Build history of the part. All positions in model axes, mm. A direction names the side the tool comes from. Round coordinates to 2 decimals unless told otherwise and drop trailing zeros. Write each loop counter-clockwise with the first axis right and the second up, starting at its lowest first coordinate (ties: lowest second). Pieces come first, ordered by that corner, then holes. Notation, with made-up numbers: M -6,54.5 L 51,54.5 A15 ccw 51,68.5 Z; hole C -23,11.5 d11. An arc over 180 degrees is marked long. One line per item, written item: value. Start each with the question number.
```python
from build123d import *

# Parameters (mm, degrees)
F0_DEPTH = 2.54
F1_R     = 38.1
F5_DEPTH = 2.541
F2_DEPTH = 25.4
F3_R     = 5.08


with BuildPart() as f0:
    # F4 (on Top) → F0 (new body)
    with BuildSketch(Plane.XY):
        with BuildLine():
            ThreePointArc((44.1325, 25.1587448763), (31.8906233853, 39.5427381462), (15.24, 48.460111432))
            ThreePointArc((15.24, 48.460111432), (0, 50.8), (-15.24, 48.460111432))
            ThreePointArc((-15.24, 48.460111432), (-31.8906233853, 39.5427381462), (-44.1325, 25.1587448763))
            ThreePointArc((-44.1325, 25.1587448763), (-35.0133309687, 14.0204203753), (-31.75, 0))
            Line((-31.75, 0), (31.75, 0))
            ThreePointArc((31.75, 0), (35.0133309687, 14.0204203753), (44.1325, 25.1587448763))
        make_face()
        with BuildLine():
            Line((73.025, 30.287569645), (15.24, 48.460111432))
            ThreePointArc((15.24, 48.460111432), (31.8906233853, 39.5427381462), (44.1325, 25.1587448763))
            ThreePointArc((44.1325, 25.1587448763), (57.9506836061, 31.2612793654), (73.025, 30.287569645))
        make_face()
        with BuildLine():
            ThreePointArc((-44.1325, 25.1587448763), (-31.8906233853, 39.5427381462), (-15.24, 48.460111432))
            Line((-15.24, 48.460111432), (-73.025, 30.287569645))
            ThreePointArc((-73.025, 30.287569645), (-57.9506836061, 31.2612793654), (-44.1325, 25.1587448763))
        make_face()
        with BuildLine():
            ThreePointArc((73.025, 30.287569645), (57.9506836061, 31.2612793654), (44.1325, 25.1587448763))
            ThreePointArc((44.1325, 25.1587448763), (49.1048419201, 13.0136274728), (50.8, 0))
            ThreePointArc((50.8, 0), (49.1048419201, -13.0136274728), (44.1325, -25.1587448763))
            ThreePointArc((44.1325, -25.1587448763), (57.9506836061, -31.2612793654), (73.025, -30.287569645))
            ThreePointArc((73.025, -30.287569645), (89.0976683508, -18.7835533113), (95.25, 0))
            ThreePointArc((95.25, 0), (89.0976683508, 18.7835533113), (73.025, 30.287569645))
        make_face()
        with BuildLine():
            ThreePointArc((-50.8, 0), (-49.1048419201, 13.0136274728), (-44.1325, 25.1587448763))
            ThreePointArc((-44.1325, 25.1587448763), (-57.9506836061, 31.2612793654), (-73.025, 30.287569645))
            ThreePointArc((-73.025, 30.287569645), (-95.25, 0), (-73.025, -30.287569645))
            ThreePointArc((-73.025, -30.287569645), (-57.9506836061, -31.2612793654), (-44.1325, -25.1587448763))
            ThreePointArc((-44.1325, -25.1587448763), (-49.1048419201, -13.0136274728), (-50.8, 0))
        make_face()
        with BuildLine():
            ThreePointArc((44.1325, -25.1587448763), (35.0133309687, -14.0204203753), (31.75, 0))
            Line((31.75, 0), (-31.75, 0))
            ThreePointArc((-31.75, 0), (-35.0133309687, -14.0204203753), (-44.1325, -25.1587448763))
            ThreePointArc((-44.1325, -25.1587448763), (-31.8906233853, -39.5427381462), (-15.24, -48.460111432))
            ThreePointArc((-15.24, -48.460111432), (0, -50.8), (15.24, -48.460111432))
            ThreePointArc((15.24, -48.460111432), (31.8906233853, -39.5427381462), (44.1325, -25.1587448763))
        make_face()
        with BuildLine():
            ThreePointArc((-44.1325, -25.1587448763), (-57.9506836061, -31.2612793654), (-73.025, -30.287569645))
            Line((-73.025, -30.287569645), (-15.24, -48.460111432))
            ThreePointArc((-15.24, -48.460111432), (-31.8906233853, -39.5427381462), (-44.1325, -25.1587448763))
        make_face()
        with BuildLine():
            ThreePointArc((73.025, -30.287569645), (57.9506836061, -31.2612793654), (44.1325, -25.1587448763))
            ThreePointArc((44.1325, -25.1587448763), (31.8906233853, -39.5427381462), (15.24, -48.460111432))
            Line((15.24, -48.460111432), (73.025, -30.287569645))
        make_face()
        with BuildLine():
            ThreePointArc((50.8, 0), (49.1048419201, 13.0136274728), (44.1325, 25.1587448763))
            ThreePointArc((44.1325, 25.1587448763), (35.0133309687, 14.0204203753), (31.75, 0))
            Line((31.75, 0), (50.8, 0))
        make_face()
        with BuildLine():
            ThreePointArc((44.1325, -25.1587448763), (49.1048419201, -13.0136274728), (50.8, 0))
            Line((50.8, 0), (31.75, 0))
            ThreePointArc((31.75, 0), (35.0133309687, -14.0204203753), (44.1325, -25.1587448763))
        make_face()
        with BuildLine():
            Line((-31.75, 0), (-50.8, 0))
            ThreePointArc((-50.8, 0), (-49.1048419201, -13.0136274728), (-44.1325, -25.1587448763))
            ThreePointArc((-44.1325, -25.1587448763), (-35.0133309687, -14.0204203753), (-31.75, 0))
        make_face()
        with BuildLine():
            ThreePointArc((-31.75, 0), (-35.0133309687, 14.0204203753), (-44.1325, 25.1587448763))
            ThreePointArc((-44.1325, 25.1587448763), (-49.1048419201, 13.0136274728), (-50.8, 0))
            Line((-50.8, 0), (-31.75, 0))
        make_face()
    extrude(amount=F0_DEPTH)

    # F1 (on face) → F5 (cut, through all)
    with BuildSketch(Plane.XY.offset(2.54)):
        Circle(F1_R)
    extrude(amount=-F5_DEPTH, mode=Mode.SUBTRACT)

    # F6 (on face) → F2 (join)
    with BuildSketch(Plane.XY.offset(2.54)):
        with BuildLine():
            Line((-73.025, -30.287569645), (-29.75025979, 23.8019335859))
            ThreePointArc((-29.75025979, 23.8019335859), (0, 38.1), (29.75025979, 23.8019335859))
            Line((29.75025979, 23.8019335859), (73.025, -30.287569645))
            ThreePointArc((73.025, -30.287569645), (95.25, 0), (73.025, 30.287569645))
            Line((73.025, 30.287569645), (15.24, 48.460111432))
            ThreePointArc((15.24, 48.460111432), (0, 50.8), (-15.24, 48.460111432))
            Line((-15.24, 48.460111432), (-73.025, 30.287569645))
            ThreePointArc((-73.025, 30.287569645), (-95.25, 0), (-73.025, -30.287569645))
        make_face()
    extrude(amount=F2_DEPTH)

    # F3
    f3_edges = [f0.edges().sort_by_distance(p)[0] for p in [
        (73.025, -30.28757, 15.24),
        (-73.025, -30.28757, 15.24),
        (-44.1325, 39.373841, 27.94),
        (-95.25, 0, 27.94),
        (-51.38763, -3.242818, 27.94),
        (0, 38.1, 27.94),
        (51.38763, -3.242818, 27.94),
        (95.25, 0, 27.94),
        (44.1325, 39.373841, 27.94),
        (0, 50.8, 27.94),
    ]]
    fillet(f3_edges, radius=F3_R)


solid = f0.part
```
Item 1: Cut at A-A, the plane x = 0. Write the cut outline in (y, z), plus the area to 3 significant figures.
Item 2: Two-plate mould, pull along X, no slides. Class faces 3 (the flat face through (-14, 42, 27.94)), 4 (the flat face through (-50.515, -2.152, 12.558)), 5 (the flat face through (-43.73, 39.5, 11.27)): pulls with the +X half, pulls with the -X half, needs draft (parallel to the pull), parting line crosses it, or undercut.
Item 3: Cut at C-C, the plane z = 25.75. Write the cut outline in (x, y).
Item 4: Drill centre lines: line 1 (Y direction, x = 0, z = 1.5); line 2 (X direction, y = 0, z = 1.8); line 3 (Z direction, x = 8, y = 42). Where is each one in solid material? Low to high.
Item 5: Drop flat-ended pins along their axis: pin 1 (6 mm diameter, centred on y = -10, z = 16.5, fed in from -X); pin 2 (8 mm diameter, centred on x = -73.5, y = -37.5, fed in from +Z); pin 3 (6 mm diameter, centred on x = -47.5, y = -27, fed in from +Z); pin 4 (1 mm diameter, centred on x = 74, z = 13.5, fed in from +Y). Give the stop position or say it passes through.
Item 6: Cut at B-B, the plane z = 17. Write the cut outline in (x, y) (3 decimals).
Item 7: Which spindle directions (+Z, -Z, +X, -X, +Y, -Y) get a long thin tool onto all of the face, cutting with end or side? Do faces 1 (the cylindrical face through (51.646, -1.247, 26.412)), 2 (the flat face through (44.537, 39.247, 11.27)). Say none if no direction does.
Computed values:
1. outline: M -50.8,0 L -38.1,0 L -38.1,2.54 L -50.8,2.54 Z; M 38.1,0 L 50.8,0 L 50.8,22.86 A5.08 ccw 45.72,27.94 L 43.18,27.94 A5.08 ccw 38.1,22.86 Z
1. area: 376 mm2
2. face 3: needs draft
2. face 4: undercut
2. face 5: pulls with the -X half
3. outline: M -76.42,-28.01 A4.18 ccw -71.41,-26.83 L -30.45,24.37 A39 cw 30.45,24.37 L 71.41,-26.83 A4.18 ccw 76.42,-28.01 A30.85 ccw 72.75,29.43 L 14.97,47.6 A49.9 ccw -14.97,47.6 L -72.75,29.43 A30.85 ccw Z
4. line 1: y = -50.8 to -38.1, 38.1 to 50.8
4. line 2: x = -95.25 to -38.1, 38.1 to 95.25
4. line 3: z = 0 to 27.92
5. pin 1: stops at x = -94.47
5. pin 2: passes through
5. pin 3: stops at z = 2.54
5. pin 4: stops at y = 30.13
6. outline: M -76.802,-28.829 A5.08 ccw -70.707,-27.39 L -29.75,23.802 A38.1 cw 29.75,23.802 L 70.707,-27.39 A5.08 ccw 76.802,-28.829 A31.75 ccw 73.025,30.288 L 15.24,48.46 A50.8 ccw -15.24,48.46 L -73.025,30.288 A31.75 ccw Z
7. face 1: +Z, -Y
7. face 2: +Z, -Z, +X, +Y
